For this review, take the finished solid that the model builds, in its own axes (mm). Face numbers are marked on the shaded views. A direction names the side the tool comes from. Round coordinates to 2 decimals unless told otherwise and drop trailing zeros. One line per item, written item: value.
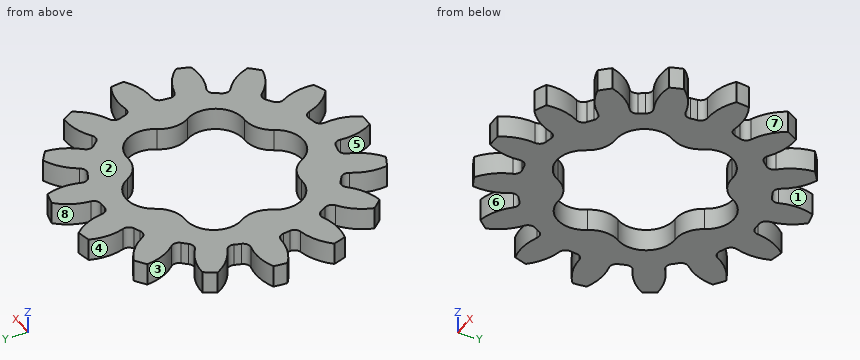
```python
from build123d import *

# Parameters (mm, degrees)
SKETCH3_R          = 21.59
GEARBODY_DEPTH     = 3.175
TOOTHCUT_DEPTH     = 4.175
CIRPATTERN1_COUNT  = 15
BOREDIA_R          = 1.499997014
BORE_DEPTH         = 12700
CUT_EXTRUDE1_DEPTH = 4.175


with BuildPart() as part:
    # Sketch3 → gearBody (new body)
    with BuildSketch(Plane.XY):
        Circle(SKETCH3_R)
    extrude(amount=GEARBODY_DEPTH)

    # Sketch2 → toothCut (cut, through all)
    with BuildSketch(Plane.XY):
        with BuildLine():
            ThreePointArc((15.776737466, -2.352729556), (15.839461945, -1.88473519), (15.888307135, -1.41508933))
            ThreePointArc((15.888307135, -1.41508933), (16.217352653, -0.757105225), (16.906558448, -0.499793338))
            ThreePointArc((16.906558448, -0.499793338), (20.511887209, 0.343917978), (23.283949955, 2.798691365))
            ThreePointArc((23.283949955, 2.798691365), (23.287267838, -2.770948491), (21.977086037, -8.184295218))
            ThreePointArc((21.977086037, -8.184295218), (19.858454824, -5.147578893), (16.551776463, -3.481408892))
            ThreePointArc((16.551776463, -3.481408892), (15.942194667, -3.069554465), (15.776737466, -2.352729556))
        make_face()
    toothcut = extrude(amount=TOOTHCUT_DEPTH, mode=Mode.SUBTRACT)

    # CirPattern1: toothCut ×15 about axis
    cirpattern1_axis = Axis((0, 0, 0), (0, 0, 1))
    for i in range(1, CIRPATTERN1_COUNT):
        add(toothcut.rotate(cirpattern1_axis, i * 360 / CIRPATTERN1_COUNT), mode=Mode.SUBTRACT)

    # boreDia → bore (cut, symmetric)
    with BuildSketch(Plane.XY):
        Circle(BOREDIA_R)
    extrude(amount=BORE_DEPTH, both=True, mode=Mode.SUBTRACT)

    # Sketch4 → Cut-Extrude1 (cut, through all)
    with BuildSketch(Plane(origin=(0, 0, 0), x_dir=(-1, 0, 0), z_dir=(0, 0, -1))):
        with BuildLine():
            ThreePointArc((-7.329682086, 8.352449747), (-5.130117272, 8.885623765), (-3.568592622, 10.523915761))
            ThreePointArc((-3.568592622, 10.523915761), (0, 12.7), (3.568592622, 10.523915761))
            ThreePointArc((3.568592622, 10.523915761), (5.130117272, 8.885623765), (7.329682086, 8.352449747))
            ThreePointArc((7.329682086, 8.352449747), (10.998522628, 6.35), (10.898274707, 2.171466014))
            ThreePointArc((10.898274707, 2.171466014), (10.260234545, 0), (10.898274707, -2.171466014))
            ThreePointArc((10.898274707, -2.171466014), (10.998522628, -6.35), (7.329682086, -8.352449747))
            ThreePointArc((7.329682086, -8.352449747), (5.130117272, -8.885623765), (3.568592622, -10.523915761))
            ThreePointArc((3.568592622, -10.523915761), (0, -12.7), (-3.568592622, -10.523915761))
            ThreePointArc((-3.568592622, -10.523915761), (-5.130117272, -8.885623765), (-7.329682086, -8.352449747))
            ThreePointArc((-7.329682086, -8.352449747), (-10.998522628, -6.35), (-10.898274707, -2.171466014))
            ThreePointArc((-10.898274707, -2.171466014), (-10.260234545, 0), (-10.898274707, 2.171466014))
            ThreePointArc((-10.898274707, 2.171466014), (-10.998522628, 6.35), (-7.329682086, 8.352449747))
        make_face()
    extrude(amount=-CUT_EXTRUDE1_DEPTH, mode=Mode.SUBTRACT)


solid = part.part
```
Item 1: For P1, Ø1, axis at x = 7, y = -6, coming from the -Z side; P2, Ø1, axis at y = 12.5, z = 0.5, coming from the -X side, all flat-tipped, find the tip position at first contact; note any pin that passes through.
Returned:
P1: through
P2: x = -11.72
Item 2: Machinability: for the marked faces 5, 6, 7 and 8, which of the approach directions +Z, -Z, +X, -X, +Y, -Y give a long, thin tool a straight path to every point of the face, cutting with its end or side? Answer none if there is none.
Returned:
face 5: +Z, -Z
face 6: +Z, -Z, -Y
face 7: +Z, -Z, +X
face 8: +Z, -Z, +Y
Item 3: Wall thickness on line 1 (Y direction, x = -7, z = 3.05); line 2 (Y direction, x = -17.5, z = 0.7); line 3 (Y direction, x = 12, z = 2.05): over which ranges is each line inside the solid? List them lowest first.
Returned:
line 1: -19.02 to -8.35, 8.35 to 14.38
line 2: -7.48 to -3.25, -0.01 to 4.17, 8.21 to 11.85
line 3: -13.9 to 10.51, 12.59 to 17.79
Item 4: The part is to be moulded in two halves that separate along X. For the marked faces 1, 2, 3 and 4, say which applies: +X half, -X half, draft (parallel to the pull), parting line (faces both ways), or undercut.
Returned:
face 1: undercut
face 2: draft
face 3: -X half
face 4: undercut
